from build123d import *

# Parameters (mm, degrees)
SKETCH_1_W          = 113
SKETCH_1_H          = 113
EXTRUDE_1_DEPTH     = 3
CUT_EXTRUDE_1_REACH = 161.834
SKETCH_2_R          = 1.7
SKETCH_3_W          = 90
SKETCH_3_H          = 105
EXTRUDE_2_DEPTH     = 2
SKETCH_5_R          = 5
EXTRUDE_3_DEPTH     = 3
CUT_EXTRUDE_2_REACH = 161.834
SKETCH_6_R          = 1.7
CUT_EXTRUDE_3_REACH = 161.834
SKETCH_7_R          = 1.7
CUT_EXTRUDE_4_REACH = 161.884
SKETCH_8_R          = 1.7
EXTRUDE_5_DEPTH     = 90
CUT_EXTRUDE_5_DEPTH = 2
SKETCH_13_W         = 2
SKETCH_13_H         = 12
EXTRUDE_6_DEPTH     = 11.5
CUT_EXTRUDE_6_REACH = 162.612
SKETCH_14_R         = 1.7
CUT_EXTRUDE_7_REACH = 164.681
EXTRUDE_7_DEPTH     = 8.5
SKETCH_17_W         = 2
SKETCH_17_H         = 11.5
EXTRUDE_8_DEPTH     = 3
FILLET_1_R          = 1
CUT_EXTRUDE_8_DEPTH = 163.681089759


with BuildPart() as part:
    # 草图1 → 凸台-拉伸1 (new body)
    with BuildSketch(Plane(origin=(0, 0, 0), x_dir=(1, 0, 0), z_dir=(0, 1, 0))):
        with Locations((56.5, 56.5)):
            Rectangle(SKETCH_1_W, SKETCH_1_H)
    extrude(amount=EXTRUDE_1_DEPTH)

    # 草图2 → 切除-拉伸1 (cut, up to next)
    with BuildSketch(Plane(origin=(0, 3, 0), x_dir=(1, 0, 0), z_dir=(0, 1, 0)), mode=Mode.PRIVATE) as cut_extrude_1_sk1:
        with Locations(Location((108.5, 69.95, 0), (0, 0, 270))):
            Circle(SKETCH_2_R)
    cut_extrude_1_tool1 = extrude(cut_extrude_1_sk1.sketch, amount=-CUT_EXTRUDE_1_REACH, mode=Mode.PRIVATE) & part.part
    # 草图2 → 切除-拉伸1 (cut, up to next)
    with BuildSketch(Plane(origin=(0, 3, 0), x_dir=(1, 0, 0), z_dir=(0, 1, 0)), mode=Mode.PRIVATE) as cut_extrude_1_sk2:
        with Locations(Location((108.5, 47.45, 0), (0, 0, 270))):
            Circle(SKETCH_2_R)
    cut_extrude_1_tool2 = extrude(cut_extrude_1_sk2.sketch, amount=-CUT_EXTRUDE_1_REACH, mode=Mode.PRIVATE) & part.part
    # 草图2 → 切除-拉伸1 (cut, up to next)
    with BuildSketch(Plane(origin=(0, 3, 0), x_dir=(1, 0, 0), z_dir=(0, 1, 0)), mode=Mode.PRIVATE) as cut_extrude_1_sk3:
        with Locations(Location((106, 30.4, 0), (0, 0, 270))):
            Circle(SKETCH_2_R)
    cut_extrude_1_tool3 = extrude(cut_extrude_1_sk3.sketch, amount=-CUT_EXTRUDE_1_REACH, mode=Mode.PRIVATE) & part.part
    # 草图2 → 切除-拉伸1 (cut, up to next)
    with BuildSketch(Plane(origin=(0, 3, 0), x_dir=(1, 0, 0), z_dir=(0, 1, 0)), mode=Mode.PRIVATE) as cut_extrude_1_sk4:
        with Locations(Location((106, 10.4, 0), (0, 0, 270))):
            Circle(SKETCH_2_R)
    cut_extrude_1_tool4 = extrude(cut_extrude_1_sk4.sketch, amount=-CUT_EXTRUDE_1_REACH, mode=Mode.PRIVATE) & part.part
    add(cut_extrude_1_tool1.solids().sort_by_distance((108.5, 3, -69.95))[0], mode=Mode.SUBTRACT)
    add(cut_extrude_1_tool2.solids().sort_by_distance((108.5, 3, -47.45))[0], mode=Mode.SUBTRACT)
    add(cut_extrude_1_tool3.solids().sort_by_distance((106, 3, -30.4))[0], mode=Mode.SUBTRACT)
    add(cut_extrude_1_tool4.solids().sort_by_distance((106, 3, -10.4))[0], mode=Mode.SUBTRACT)

    # 草图3 → 凸台-拉伸2 (add)
    with BuildSketch(Plane(origin=(0, 0, 0), x_dir=(1, 0, 0), z_dir=(0, 1, 0))):
        with Locations((55.5, 60.5)):
            Rectangle(SKETCH_3_W, SKETCH_3_H)
    extrude(amount=-EXTRUDE_2_DEPTH)

    # 草图5 → 凸台-拉伸3 (add)
    with BuildSketch(Plane.XZ):
        with Locations((79.5, -1)):
            Circle(SKETCH_5_R)
        with Locations((31.5, -1)):
            Circle(SKETCH_5_R)
    extrude(amount=-EXTRUDE_3_DEPTH)

    # 草图6 → 切除-拉伸2 (cut, up to next)
    with BuildSketch(Plane.XZ, mode=Mode.PRIVATE) as cut_extrude_2_sk1:
        with Locations(Location((31.5, -1, 0), (0, 0, 270))):
            Circle(SKETCH_6_R)
    cut_extrude_2_tool1 = extrude(cut_extrude_2_sk1.sketch, amount=-CUT_EXTRUDE_2_REACH, mode=Mode.PRIVATE) & part.part
    # 草图6 → 切除-拉伸2 (cut, up to next)
    with BuildSketch(Plane.XZ, mode=Mode.PRIVATE) as cut_extrude_2_sk2:
        with Locations(Location((79.5, -1, 0), (0, 0, 270))):
            Circle(SKETCH_6_R)
    cut_extrude_2_tool2 = extrude(cut_extrude_2_sk2.sketch, amount=-CUT_EXTRUDE_2_REACH, mode=Mode.PRIVATE) & part.part
    add(cut_extrude_2_tool1.solids().sort_by_distance((31.5, 0, -1))[0], mode=Mode.SUBTRACT)
    add(cut_extrude_2_tool2.solids().sort_by_distance((79.5, 0, -1))[0], mode=Mode.SUBTRACT)

    # 草图7 → 切除-拉伸3 (cut, up to next)
    with BuildSketch(Plane.XZ, mode=Mode.PRIVATE) as cut_extrude_3_sk1:
        with Locations(Location((5, -10.4, 0), (0, 0, 270))):
            Circle(SKETCH_7_R)
    cut_extrude_3_tool1 = extrude(cut_extrude_3_sk1.sketch, amount=-CUT_EXTRUDE_3_REACH, mode=Mode.PRIVATE) & part.part
    # 草图7 → 切除-拉伸3 (cut, up to next)
    with BuildSketch(Plane.XZ, mode=Mode.PRIVATE) as cut_extrude_3_sk2:
        with Locations(Location((5, -30.4, 0), (0, 0, 270))):
            Circle(SKETCH_7_R)
    cut_extrude_3_tool2 = extrude(cut_extrude_3_sk2.sketch, amount=-CUT_EXTRUDE_3_REACH, mode=Mode.PRIVATE) & part.part
    # 草图7 → 切除-拉伸3 (cut, up to next)
    with BuildSketch(Plane.XZ, mode=Mode.PRIVATE) as cut_extrude_3_sk3:
        with Locations(Location((5, -65.4, 0), (0, 0, 270))):
            Circle(SKETCH_7_R)
    cut_extrude_3_tool3 = extrude(cut_extrude_3_sk3.sketch, amount=-CUT_EXTRUDE_3_REACH, mode=Mode.PRIVATE) & part.part
    add(cut_extrude_3_tool1.solids().sort_by_distance((5, 0, -10.4))[0], mode=Mode.SUBTRACT)
    add(cut_extrude_3_tool2.solids().sort_by_distance((5, 0, -30.4))[0], mode=Mode.SUBTRACT)
    add(cut_extrude_3_tool3.solids().sort_by_distance((5, 0, -65.4))[0], mode=Mode.SUBTRACT)

    # 草图8 → 切除-拉伸4 (cut, up to next)
    with BuildSketch(Plane.XZ.offset(2), mode=Mode.PRIVATE) as cut_extrude_4_sk1:
        with Locations(Location((25.5, -83, 0), (0, 0, 270))):
            Circle(SKETCH_8_R)
    cut_extrude_4_tool1 = extrude(cut_extrude_4_sk1.sketch, amount=-CUT_EXTRUDE_4_REACH, mode=Mode.PRIVATE) & part.part
    # 草图8 → 切除-拉伸4 (cut, up to next)
    with BuildSketch(Plane.XZ.offset(2), mode=Mode.PRIVATE) as cut_extrude_4_sk2:
        with Locations(Location((85.5, -83, 0), (0, 0, 270))):
            Circle(SKETCH_8_R)
    cut_extrude_4_tool2 = extrude(cut_extrude_4_sk2.sketch, amount=-CUT_EXTRUDE_4_REACH, mode=Mode.PRIVATE) & part.part
    add(cut_extrude_4_tool1.solids().sort_by_distance((25.5, -2, -83))[0], mode=Mode.SUBTRACT)
    add(cut_extrude_4_tool2.solids().sort_by_distance((85.5, -2, -83))[0], mode=Mode.SUBTRACT)

    # 草图10 → 凸台-拉伸5 (add)
    with BuildSketch(Plane(origin=(100.5, 0, 0), x_dir=(0, 0, -1), z_dir=(1, 0, 0))):
        Polygon((113, 0), (116.464101615, -2), (113, -2), align=None)
    extrude(amount=-EXTRUDE_5_DEPTH)

    # 草图11 → 切除-拉伸5 (cut)
    with BuildSketch(Plane(origin=(0, -2, 0), x_dir=(1, 0, 0), z_dir=(0, 1, 0))):
        with BuildLine():
            Line((20.5, 83), (20.5, 23))
            ThreePointArc((20.5, 23), (25.5, 18), (30.5, 23))
            Line((30.5, 23), (30.5, 83))
            ThreePointArc((30.5, 83), (25.5, 88), (20.5, 83))
        make_face()
        with BuildLine():
            Line((80.5, 83), (80.5, 23))
            ThreePointArc((80.5, 23), (85.5, 18), (90.5, 23))
            Line((90.5, 23), (90.5, 83))
            ThreePointArc((90.5, 83), (85.5, 88), (80.5, 83))
        make_face()
    extrude(amount=CUT_EXTRUDE_5_DEPTH, mode=Mode.SUBTRACT)

    # 草图13 → 凸台-拉伸6 (add)
    with BuildSketch(Plane.XZ):
        with Locations((4, -83)):
            Rectangle(SKETCH_13_W, SKETCH_13_H)
    extrude(amount=EXTRUDE_6_DEPTH)

    # 草图14 → 切除-拉伸6 (cut, up to next)
    with BuildSketch(Plane.ZY.offset(-3), mode=Mode.PRIVATE) as cut_extrude_6_sk1:
        with Locations((-83.5, -5)):
            Circle(SKETCH_14_R)
    cut_extrude_6_tool1 = extrude(cut_extrude_6_sk1.sketch, amount=-CUT_EXTRUDE_6_REACH, mode=Mode.PRIVATE) & part.part
    add(cut_extrude_6_tool1.solids().sort_by_distance((3, -5, -83.5))[0], mode=Mode.SUBTRACT)

    # 草图15 → 切除-拉伸7 (cut, up to next)
    with BuildSketch(Plane.XZ, mode=Mode.PRIVATE) as cut_extrude_7_sk1:
        Polygon((113, -100.875644347), (106, -113), (113, -113), align=None)
    cut_extrude_7_tool1 = extrude(cut_extrude_7_sk1.sketch, amount=-CUT_EXTRUDE_7_REACH, mode=Mode.PRIVATE) & part.part
    add(cut_extrude_7_tool1.solids().sort_by_distance((110.666667, 0, -108.958548))[0], mode=Mode.SUBTRACT)

    # 草图16 → 凸台-拉伸7 (add)
    with BuildSketch(Plane.XZ):
        Polygon((113, -99.5), (107.5, -99.5), (107.5, -110.401923789), (113, -100.875644347), align=None)
    extrude(amount=EXTRUDE_7_DEPTH)

    # 草图17 → 凸台-拉伸8 (add)
    with BuildSketch(Plane.ZY.offset(-3)):
        with Locations((-78, -5.75)):
            Rectangle(SKETCH_17_W, SKETCH_17_H)
    extrude(amount=EXTRUDE_8_DEPTH)

    # 圆角1
    fillet_1_edges = [part.edges().sort_by_distance(p)[0] for p in [
        (3, -5.75, -79),
    ]]
    fillet(fillet_1_edges, radius=FILLET_1_R)

    # 草图19 → 切除-拉伸8 (cut, through all)
    with BuildSketch(Plane.ZY):
        Polygon((-113, 0), (-107.803847577, 3), (-113, 3), align=None)
    extrude(amount=-CUT_EXTRUDE_8_DEPTH, mode=Mode.SUBTRACT)


solid = part.part
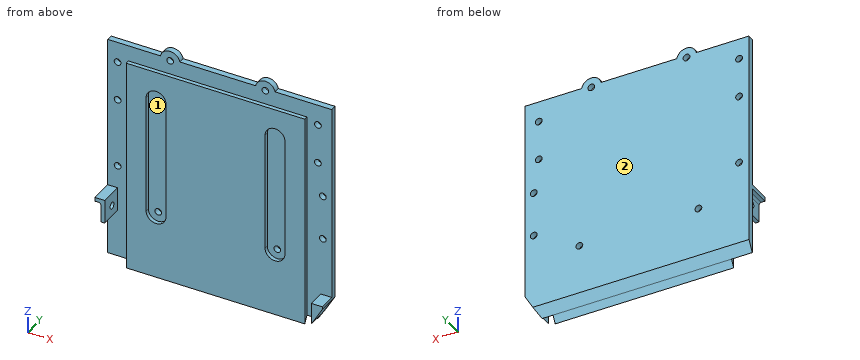
Model file for the job. Use its own axes, mm. Face numbers are marked on the shaded views. Coordinates: 2 decimals unless noted, no trailing zeros. Order: outer loops, then holes, each group sorted by start corner. A loop starts at its lowest first (then second) coordinate and runs counter-clockwise, first axis right, second up. Notation, with made-up numbers: M 62.5,77 L 110.5,77 A24 ccw 110.5,99 Z; hole C 23.5,72 d8. An arc over 180 degrees is marked long. Return JSON: item names as keys, results as strings.
1. Drill centre lines: probe 1 along X at (y, z) = (1, -1); probe 2 along X at (y, z) = (1.8, -30.4); probe 3 along X at (y, z) = (1.2, -47.45). Where is each one in solid material? Low to high.
Ans:
{"probe 1": "0 to 29.8, 33.2 to 77.8, 81.2 to 113", "probe 2": "0 to 3.3, 6.7 to 104.3, 107.7 to 113", "probe 3": "0 to 106.8, 110.2 to 113"}
2. Saw through at A-A (y = -5). Give the cut face in (x, z), and give its area (3 significant figures).
Ans:
{"outline": "M 0,-79 L 2,-79 A1 cw 3,-80 L 3,-81.8 L 5,-81.8 L 5,-77 L 0,-77 Z; M 3,-89 L 5,-89 L 5,-85.2 L 3,-85.2 Z; M 107.5,-110.4 L 113,-100.88 L 113,-99.5 L 107.5,-99.5 Z", "area": "57.2 mm^2"}
3. Saw through at C-C (z = -65.4). Give the cut face in (x, y).
Ans:
{"outline": "M 0,0 L 3.3,0 L 3.3,3 L 0,3 Z; M 6.7,0 L 10.5,0 L 10.5,-2 L 20.5,-2 L 20.5,0 L 30.5,0 L 30.5,-2 L 80.5,-2 L 80.5,0 L 90.5,0 L 90.5,-2 L 100.5,-2 L 100.5,0 L 113,0 L 113,3 L 6.7,3 Z"}
4. Pull direction Z, two halves, no side cores. Call the marked faces 1 and 2: +Z half, -Z half, draft (parallel to the pull), parting line (faces both ways), or undercut.
Ans:
{"face 1": "undercut", "face 2": "draft"}
5. Saw through at B-B (z = -30.4). Give the cut face in (x, y).
Ans:
{"outline": "M 0,0 L 3.3,0 L 3.3,3 L 0,3 Z; M 6.7,0 L 10.5,0 L 10.5,-2 L 20.5,-2 L 20.5,0 L 30.5,0 L 30.5,-2 L 80.5,-2 L 80.5,0 L 90.5,0 L 90.5,-2 L 100.5,-2 L 100.5,0 L 104.3,0 L 104.3,3 L 6.7,3 Z; M 107.7,0 L 113,0 L 113,3 L 107.7,3 Z"}
6. Saw through at D-D (x = 94). Give the cut face in (y, z).
Ans:
{"outline": "M -2,-116.46 L 3,-107.8 L 3,0 L 0,0 L 0,-8 L -2,-8 Z"}
7. Flat gauge pins, fed straight in: pin 1 (4 mm diameter, centred on x = 85.5, z = -83, fed in from -Y); pin 2 (1.6 mm diameter, centred on y = -1, z = -38, fed in from +X); pin 3 (4.5 mm diameter, centred on y = -5, z = -83.5, fed in from -X). Where does each tip first touch, or does it go through?
Ans:
{"pin 1": "y = 0", "pin 2": "x = 100.5", "pin 3": "x = 3"}
